from build123d import *

# Parameters (mm, degrees)
BOSS_EXTRUDE1_DEPTH = 25
SKETCH3_W           = 9
SKETCH3_H           = 3
TAPPED_HOLE1_D      = 4.2
TAPPED_HOLE1_DEPTH  = 14
TAPPED_HOLE1_TIP    = 1.2618073
FILLET1_R           = 0.5


with BuildPart() as part:
    # Sketch1 → Boss-Extrude1 (new body)
    with BuildSketch(Plane(origin=(0, 0, 0), x_dir=(0, 0, -1), z_dir=(1, 0, 0))):
        Polygon((0, 5.773502692), (-5, 2.886751346), (-5, -2.886751346), (0, -5.773502692), (5, -2.886751346), (5, 2.886751346), align=None)
    extrude(amount=BOSS_EXTRUDE1_DEPTH)

    # Sketch2 → Cut-Revolve1 (revolve, cut)
    with BuildSketch(Plane.XY):
        Polygon((0.446581987, 5.773502692), (0, 5.773502692), (0, 5), align=None)
        Polygon((25, 5), (25, 5.773502692), (24.553418013, 5.773502692), align=None)
    revolve(axis=Axis((0, 0, 0), (1, 0, 0)), mode=Mode.SUBTRACT)

    # Sketch3 → Revolve1 (revolve)
    with BuildSketch(Plane.XY):
        with Locations((-4.5, 1.5)):
            Rectangle(SKETCH3_W, SKETCH3_H)
    revolve(axis=Axis((0, 0, 0), (-1, 0, 0)))

    # Tapped Hole1
    with Locations(Plane(origin=(25, 0, 0), x_dir=(0, 0, -1), z_dir=(1, 0, 0))):
        with Locations((0, 0)):
            Hole(TAPPED_HOLE1_D / 2, depth=TAPPED_HOLE1_DEPTH)
            with Locations((0, 0, -(TAPPED_HOLE1_DEPTH + TAPPED_HOLE1_TIP / 2))):  # 118° drill point
                Cone(0, TAPPED_HOLE1_D / 2, TAPPED_HOLE1_TIP, mode=Mode.SUBTRACT)

    # Fillet1
    fillet1_edges = [part.edges().sort_by_distance(p)[0] for p in [
        (0, -3, 0),
    ]]
    fillet(fillet1_edges, radius=FILLET1_R)


solid = part.part
Work out the finished part from the listing and answer in its coordinate system (mm). A direction names the side the tool comes from. Round coordinates to 2 decimals unless told otherwise and drop trailing zeros. Write each loop counter-clockwise with the first axis right and the second up, starting at its lowest first coordinate (ties: lowest second). Pieces come first, ordered by that corner, then holes.
1) The mould has two halves that part along Y. Classify faces 1 (the conical face through (9.96, 0.11, -0.35)), 2 (the conical face through (24.894, -2.603, -4.483)), 3 (the flat face through (12, 0, 5)), 4 (the conical face through (24.894, 5.184, -0.013)): pulls with the +Y half, pulls with the -Y half, needs draft (parallel to the pull), parting line crosses it, or undercut.
2) Given pin 1 Ø2 at (x, z) = (4, 1.5) entering from -Y; pin 2 Ø4 at (x, z) = (4, 1) entering from -Y; pin 3 Ø2 at (x, z) = (-4.5, -2) entering from -Y, each flat-ended and moving along its own axis, determine where each tip first touches the part or whether it passes through.
3) A cutting plane is placed at A-A (x = 22). Give the vertices of the cut face in (y, z), plus the area to 3 significant figures.
4) Straight lines are drawn through the part: line 1 (Z direction, x = 18.25, y = 0); line 2 (X direction, y = 2, z = -4); line 3 (Y direction, x = 13, z = 1.5). For each, find the intervals that lie inside material, in ascending order.
5) A tool of negligible diameter and unlimited length cuts with its end or side. For faces 5 (the flat face through (0, -3.3, -2.2)), 6 (the conical face through (0.11, 2.6, 4.49)), from which of +Z, -Z, +X, -X, +Y, -Y can it reach the whole face along a straight path? Write none if from no direction.
6) A cutting plane is placed at B-B (x = -2). Give the vertices of the cut face in (y, z), plus the area to 3 significant figures.
Completed:
1. face 1: undercut
1. face 2: pulls with the -Y half
1. face 3: needs draft
1. face 4: pulls with the +Y half
2. pin 1: stops at y = -5.48
2. pin 2: stops at y = -5.77
2. pin 3: stops at y = -2.83
3. outline: (-5.77, 0) - (-2.89, -5) - (2.89, -5) - (5.77, 0) - (2.89, 5) - (-2.89, 5) - close; hole circle Ø4.2 at (0, 0)
3. area: 72.7 mm2
4. line 1: z = -5 to -2.1, 2.1 to 5
4. line 2: x = 0 to 25
4. line 3: y = -4.91 to -1.47, 1.47 to 4.91
5. face 5: -X
5. face 6: +Z, -X, +Y
6. outline: circle Ø6 at (0, 0)
6. area: 28.3 mm2
